Design review of the part built by this model. Coordinates are the model's own, in mm. A direction names the side the tool comes from. Give positions to 0.01 mm unless a question says otherwise; leave off trailing zeros. Order: outer loops, then holes, each group sorted by start corner. A loop starts at its lowest first (then second) coordinate and runs counter-clockwise, first axis right, second up. Notation, with made-up numbers: (35.25, 58.5) -> (64.25, 58.5) arc R16 cw to (64.25, 75.5) -> close; hole circle Ø6 at (16, 45.5). An arc over 180 degrees is marked (long way). Return JSON: item names as keys, results as strings.
```python
from build123d import *

# Parameters (mm, degrees)
BASE_DEPTH           = 5
BOARDSLOT_DEPTH      = 45.86446744
BOARDSLOT_DEPTH_BACK = 45.86446744
SUPPORTMOUNT_DEPTH   = 5
BOSS_EXTRUDE1_DEPTH  = 1
SKETCH10_W           = 20
SKETCH10_H           = 2
BOSS_EXTRUDE2_DEPTH  = 2.5
CHAMFER1_SIZE        = 1


with BuildPart() as part:
    # Sketch1 → Base (new body)
    with BuildSketch(Plane(origin=(0, 0, 0), x_dir=(1, 0, 0), z_dir=(0, 1, 0))):
        with BuildLine():
            Line((-24.330127019, -2.5), (-2.165063509, 35.891016151))
            ThreePointArc((-2.165063509, 35.891016151), (0, 37.141016151), (2.165063509, 35.891016151))
            Line((2.165063509, 35.891016151), (24.330127019, -2.5))
            ThreePointArc((24.330127019, -2.5), (23.415063509, -5.915063509), (20, -5))
            Line((20, -5), (2.165063509, 25.891016151))
            ThreePointArc((2.165063509, 25.891016151), (0, 27.141016151), (-2.165063509, 25.891016151))
            Line((-2.165063509, 25.891016151), (-20, -5))
            ThreePointArc((-20, -5), (-23.415063509, -5.915063509), (-24.330127019, -2.5))
        make_face()
    extrude(amount=BASE_DEPTH)

    # Sketch2 → BoardSlot (cut, two sides: drawn at the far end of the back side and taken through both)
    with BuildSketch(Plane(origin=(0, 0, 0), x_dir=(0, 0, -1), z_dir=(1, 0, 0)).offset(-BOARDSLOT_DEPTH_BACK)):
        Polygon((-1.481783147, 2.110540039), (-0.610225719, 12.07248702), (1.481783147, 11.889459961), (0.610225719, 1.92751298), align=None)
        Polygon((3.389774281, 12.07248702), (5.481783147, 11.889459961), (4.610225719, 1.92751298), (2.518216853, 2.110540039), align=None)
        Polygon((7.389774281, 12.07248702), (9.481783147, 11.889459961), (8.610225719, 1.92751298), (6.518216853, 2.110540039), align=None)
        Polygon((11.389774281, 12.07248702), (13.481783147, 11.889459961), (12.610225719, 1.92751298), (10.518216853, 2.110540039), align=None)
        Polygon((15.389774281, 12.07248702), (17.481783147, 11.889459961), (16.610225719, 1.92751298), (14.518216853, 2.110540039), align=None)
    extrude(amount=BOARDSLOT_DEPTH + BOARDSLOT_DEPTH_BACK, mode=Mode.SUBTRACT)

    # Sketch3 → SupportMount (add)
    with BuildSketch(Plane(origin=(0, 0, 0), x_dir=(1, 0, 0), z_dir=(0, 1, 0))):
        with BuildLine():
            Line((5.906733437, 29.410253733), (2.165063509, 35.891016151))
            ThreePointArc((2.165063509, 35.891016151), (0, 37.141016151), (-2.165063509, 35.891016151))
            Line((-2.165063509, 35.891016151), (-5.906733437, 29.410253733))
            ThreePointArc((-5.906733437, 29.410253733), (0, 19.179491924), (5.906733437, 29.410253733))
        make_face()
    extrude(amount=SUPPORTMOUNT_DEPTH)

    # Sketch9 → Boss-Extrude1 (add, symmetric)
    with BuildSketch(Plane(origin=(0, 0, 0), x_dir=(0, 0, -1), z_dir=(1, 0, 0))):
        with BuildLine():
            Line((21.217819535, 0), (37.217819535, 0))
            ThreePointArc((37.217819535, 0), (40.04624666, 1.171572875), (41.217819535, 4))
            Line((41.217819535, 4), (41.217819535, 16))
            ThreePointArc((41.217819535, 16), (40.04624666, 18.828427125), (37.217819535, 20))
            Line((37.217819535, 20), (25.217819535, 20))
            ThreePointArc((25.217819535, 20), (22.38939241, 18.828427125), (21.217819535, 16))
            Line((21.217819535, 16), (21.217819535, 0))
        make_face()
    extrude(amount=BOSS_EXTRUDE1_DEPTH, both=True)

    # Sketch10 → Boss-Extrude2 (add, symmetric)
    with BuildSketch(Plane(origin=(0, 0, 0), x_dir=(0, 0, -1), z_dir=(1, 0, 0))):
        with Locations((31.217819535, 15)):
            Rectangle(SKETCH10_W, SKETCH10_H)
        with Locations((31.217819535, 10)):
            Rectangle(SKETCH10_W, SKETCH10_H)
    extrude(amount=BOSS_EXTRUDE2_DEPTH, both=True)

    # Chamfer1
    chamfer1_edges = [part.edges().sort_by_distance(p)[0] for p in [
        (-2.5, 9, -31.217819535),
        (-2.5, 11, -31.217819535),
        (-2.5, 14, -31.217819535),
        (-2.5, 16, -31.217819535),
        (2.5, 9, -31.217819535),
        (2.5, 11, -31.217819535),
        (2.5, 14, -31.217819535),
        (2.5, 16, -31.217819535),
    ]]
    chamfer(chamfer1_edges, length=CHAMFER1_SIZE - 0.0001)  # a hair under: the kernel refuses the full size


solid = part.part
```
Item 1: Machinability: for faces 1 (the face through (17.219, 3.485, -4.747)), 2 (the face through (18.432, 3.535, -2.643)), 3 (the face through (1, 13, -31)), which of the approach directions +Z, -Z, +X, -X, +Y, -Y give a long, thin tool a straight path to every point of the face, cutting with its end or side? Answer none if there is none.
Result set:
{"face 1": "+X, -X, +Y", "face 2": "+X, -X", "face 3": "+Z, -Z, +X"}
Item 2: Add section C-C (x = 4). Give the boundary of the cut face in (y, z), plus the area to 3 significant figures.
Result set:
{"outline": "(0, -32.71) -> (5, -32.71) -> (5, -20.48) -> (0, -20.48) -> close", "area": "61.2 mm^2"}
Item 3: For pin 1 (1.5 mm diameter, centred on x = 12.5, z = -14, fed in from +Y); pin 2 (1 mm diameter, centred on y = 4, z = -27, fed in from -X); pin 3 (10 mm diameter, centred on x = 14.5, y = 8, fed in from +Z), all flat-tipped, find the tip position at first contact; note any pin that passes through.
Result set:
{"pin 1": "stops at y = 5", "pin 2": "stops at x = -7.59", "pin 3": "stops at z = 2.4"}
Item 4: Add section A-A (z = 3.75). Give the boundary of the cut face in (x, y).
Result set:
{"outline": "(-24.67, 0) -> (-19.28, 0) -> (-19.28, 5) -> (-24.67, 5) -> close; (19.28, 0) -> (24.67, 0) -> (24.67, 5) -> (19.28, 5) -> close"}
Item 5: Mouldability with a two-part tool opening along Y and no side actions: class faces 4 (the face through (23.46, 2.46, 5.89)), 5 (the face through (-16.205, 3.535, -6.643)), 6 (the face through (-19, 5, -2)) as released by +Y, released by -Y, zero draft, split by the parting line, or undercut.
Result set:
{"face 4": "zero draft", "face 5": "undercut", "face 6": "released by +Y"}
Item 6: Add section D-D (y = 7.5). Give the boundary of the cut face in (x, z).
Result set:
{"outline": "(-1, -41.22) -> (1, -41.22) -> (1, -21.22) -> (-1, -21.22) -> close"}
Item 7: Wall thickness on L1, parallel to X at y = 13.75, z = -28.5; L2, parallel to Y at x = 1, z = -21; L3, parallel to Z at x = 9, y = 3: over which ranges is each line inside the solid? List them lowest first. Write a range as [from, to].
Result set:
{"L1": "x = [-1, 1]", "L2": "y = [0, 5]", "L3": "z = [-24.05, -16.7], [-14.6, -14.05]"}
